Model file for the job. Use its own axes, mm. A direction names the side the tool comes from. Round coordinates to 2 decimals unless told otherwise and drop trailing zeros. Write each loop counter-clockwise with the first axis right and the second up, starting at its lowest first coordinate (ties: lowest second). Pieces come first, ordered by that corner, then holes. Notation, with made-up numbers: (10.5, -40) - (19.5, -40) arc R19 ccw to (19.5, -21) - close; hole circle Ø11 at (-39, 87.25). An arc over 180 degrees is marked (long way). One line per item, written item: value.
from build123d import *

# Parameters (mm, degrees)
F1_DEPTH = 500.5
F2_W     = 10
F2_H     = 10
F3_DEPTH = 1
F4_W     = 1
F4_H     = 1
F5_DEPTH = 505.5


with BuildPart() as f1:
    # F0 (on Top) → F1 (new body)
    with BuildSketch(Plane.XY):
        Polygon((5, 15.438399), (-5, 15.438399), (-5, 14.438399), (-3.67, 14.438399), (-3.67, -1.142601), (-5, -1.142601), (-5, -2.142601), (5, -2.142601), (5, -1.142601), (3.67, -1.142601), (3.67, 14.438399), (5, 14.438399), align=None)
    extrude(amount=F1_DEPTH)

    # F2 (on face) → F3 (join)
    with BuildSketch(Plane.XZ.offset(2.142601)):
        with Locations((0, 5)):
            Rectangle(F2_W, F2_H)
    extrude(amount=F3_DEPTH)

    # F4 (on face) → F5 (cut)
    with BuildSketch(Plane.XY.offset(500.5)):
        with Locations((-2.47, 12.938399)):
            Rectangle(F4_W, F4_H)
        with Locations((-2.47, 0.357399)):
            Rectangle(F4_W, F4_H)
        with Locations((2.47, 12.938399)):
            Rectangle(F4_W, F4_H)
        with Locations((2.47, 0.357399)):
            Rectangle(F4_W, F4_H)
        with Locations((-2.47, 6.678488)):
            Rectangle(F4_W, F4_H)
        with Locations((2.47, 6.678488)):
            Rectangle(F4_W, F4_H)
        with Locations((-2.47, 11.044263)):
            Rectangle(F4_W, F4_H)
        with Locations((2.47, 11.044263)):
            Rectangle(F4_W, F4_H)
        with Locations((-2.47, 2.251399)):
            Rectangle(F4_W, F4_H)
        with Locations((2.47, 2.251399)):
            Rectangle(F4_W, F4_H)
    extrude(amount=-F5_DEPTH, mode=Mode.SUBTRACT)


solid = f1.part
1. Wall check: probe 1 along Y at (x, z) = (-2.75, 418); probe 2 along X at (y, z) = (11.5, 158); probe 3 along Y at (x, z) = (-3.75, 247.5). Give the ranges that are in metal, low to high. Write a range as [from, to].
Report:
probe 1: [-2.14, -0.14], [0.86, 1.75], [2.75, 6.18], [7.18, 10.54], [11.54, 12.44], [13.44, 15.44]
probe 2: [-3.67, -2.97], [-1.97, 1.97], [2.97, 3.67]
probe 3: [-2.14, -1.14], [14.44, 15.44]
2. Band-saw the part on B-B on x = 0. Write the cut outline in (y, z), plus the area to 3 significant figures.
Report:
outline: (-3.14, 0) - (15.44, 0) - (15.44, 500.5) - (-2.14, 500.5) - (-2.14, 10) - (-3.14, 10) - close
area: 8,810 mm²
3. Drop flat-ended pins along their axis: pin 1 (3 mm diameter, centred on y = 6.5, z = 72.5, fed in from -X); pin 2 (6 mm diameter, centred on x = -2.5, z = 144, fed in from -Y); pin 3 (5 mm diameter, centred on y = 2.5, z = 147.5, fed in from +X); pin 4 (2 mm diameter, centred on x = 2.5, y = 7, fed in from -Z). Give the stop position or say it passes through.
Report:
pin 1: x = -3.67
pin 2: y = -2.14
pin 3: x = 3.67
pin 4: z = 0
4. Mould opens along Y. For faces 3 (the face through (0, 7, 500.5)), 4 (the face through (0, -3.143, 5)), 5 (the face through (-3.67, 7, 247)), 6 (the face through (3.67, 7, 247)) say: released by +Y, released by -Y, zero draft, split by the parting line, or undercut.
Report:
face 3: zero draft
face 4: released by -Y
face 5: undercut
face 6: undercut
5. Tool access for faces 1 (the face through (0, 15.438, 247)), 2 (the face through (0, -2.143, 252)): list every direction of +Z, -Z, +X, -X, +Y, -Y with a clear straight run to the whole face (end or side of a thin tool).
Report:
face 1: +Z, -Z, +X, -X, +Y
face 2: +Z, +X, -X, -Y
6. Band-saw the part on A-A on z = 245. State how many separate pieces and enclosed holes the cut face has, plus the area to 3 significant figures.
Report:
separate pieces: 1
enclosed holes: 10
area: 124 mm²
